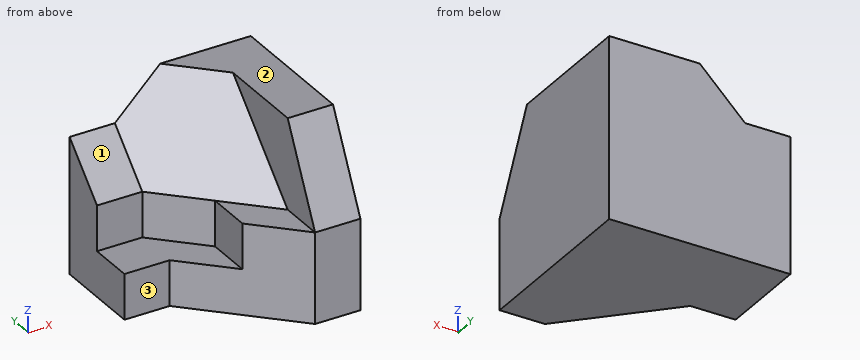
```python
from build123d import *

# Parameters (mm, degrees)
SKETCH1_W            = 40
SKETCH1_H            = 40
BOSS_EXTRUDE1_DEPTH  = 20
CUT_EXTRUDE1_DEPTH   = 20
SKETCH3_W            = 10
SKETCH3_H            = 10
CUT_EXTRUDE2_DEPTH   = 10
BOSS_EXTRUDE2_DEPTH  = 10
BOSS_EXTRUDE3_DEPTH  = 29
BOSS_EXTRUDE4_DEPTH  = 10
CUT_EXTRUDE3_DEPTH   = 10
BOSS_EXTRUDE5_DEPTH  = 10
SKETCH17_W           = 10
SKETCH17_H           = 10
BOSS_EXTRUDE8_DEPTH  = 30
CUT_EXTRUDE4_DEPTH   = 30
CUT_EXTRUDE5_DEPTH   = 10
CUT_EXTRUDE6_DEPTH   = 10
SKETCH21_W           = 5
SKETCH21_H           = 10
BOSS_EXTRUDE9_DEPTH  = 5
CUT_EXTRUDE7_DEPTH   = 5
CUT_EXTRUDE8_DEPTH   = 5
CUT_EXTRUDE9_DEPTH   = 5
BOSS_EXTRUDE10_DEPTH = 5
BOSS_EXTRUDE11_DEPTH = 5
SKETCH27_W           = 20
SKETCH27_H           = 5
BOSS_EXTRUDE12_DEPTH = 40
CUT_EXTRUDE10_DEPTH  = 19


with BuildPart() as part:
    # Sketch1 → Boss-Extrude1 (new body)
    with BuildSketch(Plane.XY):
        with Locations((20, 20)):
            Rectangle(SKETCH1_W, SKETCH1_H)
    extrude(amount=BOSS_EXTRUDE1_DEPTH)

    # Sketch2 → Cut-Extrude1 (cut)
    with BuildSketch(Plane.XY.offset(20)):
        Polygon((0, 0), (30, 0), (10, 20), (0, 20), align=None)
    extrude(amount=-CUT_EXTRUDE1_DEPTH, mode=Mode.SUBTRACT)

    # Sketch3 → Cut-Extrude2 (cut)
    with BuildSketch(Plane.ZY):
        with Locations((15, 25)):
            Rectangle(SKETCH3_W, SKETCH3_H)
    extrude(amount=-CUT_EXTRUDE2_DEPTH, mode=Mode.SUBTRACT)

    # Sketch5 → Boss-Extrude2 (add)
    with BuildSketch(Plane(origin=(40, 0, 0), x_dir=(0, 0, -1), z_dir=(1, 0, 0))):
        Polygon((-20, 40), (-20, 0), (-40, 10), (-40, 40), align=None)
    extrude(amount=-BOSS_EXTRUDE2_DEPTH)

    # Sketch7 → Boss-Extrude3 (add)
    with BuildSketch(Plane.XY.offset(40)):
        Polygon((30, 30), (30, 40), (20, 40), align=None)
    extrude(amount=-BOSS_EXTRUDE3_DEPTH)

    # Sketch8 → Boss-Extrude4 (add)
    with BuildSketch(Plane.ZY):
        Polygon((20, 40), (20, 30), (30, 40), align=None)
    extrude(amount=-BOSS_EXTRUDE4_DEPTH)

    # Sketch9 → Cut-Extrude3 (cut)
    with BuildSketch(Plane.XY.offset(20)):
        Polygon((10, 30), (20, 20), (20, 10), (10, 20), align=None)
    extrude(amount=-CUT_EXTRUDE3_DEPTH, mode=Mode.SUBTRACT)

    # Sketch15 → Boss-Extrude5 (add)
    with BuildSketch(Plane(origin=(6.666666667, 6.666666667, -6.666666667), x_dir=(-0.40824829046386313, -0.40824829046386274, -0.8164965809277261), z_dir=(0.5773502691896262, 0.5773502691896255, -0.5773502691896256))):
        Polygon((-57.154760665, 0), (-57.154760665, 14.142135624), (-32.659863237, 14.142135624), (-32.659863237, -14.142135624), align=None)
    extrude(amount=BOSS_EXTRUDE5_DEPTH)

    # Sketch17 → Boss-Extrude8 (add)
    with BuildSketch(Plane.ZY):
        with Locations((25, 35)):
            Rectangle(SKETCH17_W, SKETCH17_H)
    extrude(amount=-BOSS_EXTRUDE8_DEPTH)

    # Sketch18 → Cut-Extrude4 (cut)
    with BuildSketch(Plane(origin=(0, 40, 0), x_dir=(1, 0, 0), z_dir=(0, 1, 0))):
        Polygon((20, -40), (31.547005384, -34.226497308), (20, -22.679491924), (20, -30), align=None)
    extrude(amount=CUT_EXTRUDE4_DEPTH, mode=Mode.SUBTRACT)

    # Sketch19 → Cut-Extrude5 (cut)
    with BuildSketch(Plane.ZY):
        Polygon((30, 40), (20, 30), (30, 30), align=None)
    extrude(amount=-CUT_EXTRUDE5_DEPTH, mode=Mode.SUBTRACT)

    # Sketch20 → Cut-Extrude6 (cut)
    with BuildSketch(Plane(origin=(6.666666667, 6.666666667, -6.666666667), x_dir=(0.40824829046386324, 0.4082482904638628, 0.816496580927726), z_dir=(-0.5773502691896261, -0.5773502691896254, 0.5773502691896257))):
        Polygon((44.907311951, 7.071067812), (44.907311951, 14.142135624), (32.659863237, 14.142135624), align=None)
    extrude(amount=CUT_EXTRUDE6_DEPTH, mode=Mode.SUBTRACT)

    # Sketch21 → Boss-Extrude9 (add)
    with BuildSketch(Plane(origin=(0, 40, 0), x_dir=(1, 0, 0), z_dir=(0, 1, 0))):
        with Locations((17.5, -35)):
            Rectangle(SKETCH21_W, SKETCH21_H)
    extrude(amount=-BOSS_EXTRUDE9_DEPTH)

    # Sketch22 → Cut-Extrude7 (cut)
    with BuildSketch(Plane(origin=(0, 40, 0), x_dir=(1, 0, 0), z_dir=(0, 1, 0))):
        Polygon((20, -40), (15, -35), (15, -40), align=None)
    extrude(amount=-CUT_EXTRUDE7_DEPTH, mode=Mode.SUBTRACT)

    # Sketch23 → Cut-Extrude8 (cut)
    with BuildSketch(Plane(origin=(6.666666667, 6.666666667, -6.666666667), x_dir=(0.40824829046386324, 0.4082482904638628, 0.816496580927726), z_dir=(-0.5773502691896261, -0.5773502691896254, 0.5773502691896257))):
        Polygon((44.907311951, 14.142135624), (44.907311951, 21.213203436), (32.659863237, 14.142135624), align=None)
    extrude(amount=CUT_EXTRUDE8_DEPTH, mode=Mode.SUBTRACT)


with BuildPart() as cut_extrude8_piece_1:
    # of the separate pieces the step leaves, piece 1, a body of its own (cut_extrude8_pieces)
    add(part.part.solids().sort_by_distance((30, 0, 0))[0])

    # Sketch25 → Boss-Extrude10 (add)
    with BuildSketch(Plane(origin=(0, 40, 0), x_dir=(1, 0, 0), z_dir=(0, 1, 0))):
        Polygon((15, -35), (10, -30), (15, -30), align=None)
    extrude(amount=-BOSS_EXTRUDE10_DEPTH)

    # Sketch26 → Boss-Extrude11 (add)
    with BuildSketch(Plane(origin=(0, 0, 30), x_dir=(-1, 0, 0), z_dir=(0, 0, -1))):
        Polygon((-15, 35), (-10, 40), (-10, 35), align=None)
    extrude(amount=BOSS_EXTRUDE11_DEPTH)

    # Sketch27 → Boss-Extrude12 (add)
    with BuildSketch(Plane(origin=(0, 0, 0), x_dir=(-1, 0, 0), z_dir=(0, 0, -1))):
        with Locations((-30, 37.5)):
            Rectangle(SKETCH27_W, SKETCH27_H)
    extrude(amount=-BOSS_EXTRUDE12_DEPTH)

    # 3DSketch1 → Cut-Extrude10 (cut, along a direction that is not the sketch's normal)
    with BuildSketch(Plane(origin=(10, 30, 20), x_dir=(0.7071067811865477, 0, 0.7071067811865475), z_dir=(0.5773502691896258, 0.5773502691896254, -0.5773502691896261))):
        Polygon((0, 0), (7.071067812, -12.247448714), (21.213203436, -12.247448714), (28.284271247, 0), (14.142135624, 24.494897428), align=None)
    extrude(amount=-CUT_EXTRUDE10_DEPTH, dir=(0, 0, -1), mode=Mode.SUBTRACT)


with BuildPart() as cut_extrude8_piece_2:
    # of the separate pieces the step leaves, piece 2, a body of its own (cut_extrude8_pieces)
    add(part.part.solids().sort_by_distance((10, 30, 30))[0])

    # Sketch24 → Cut-Extrude9 (cut)
    with BuildSketch(Plane(origin=(3.779915321, 3.779915321, -3.779915321), x_dir=(-0.4082482904638635, -0.40824829046386263, -0.816496580927726), z_dir=(0.5773502691896261, 0.5773502691896255, -0.5773502691896258))):
        Polygon((-41.371778045, 14.142135624), (-41.371778045, 15.089479079), (-39.730931049, 14.142135624), align=None)
    extrude(amount=-CUT_EXTRUDE9_DEPTH, mode=Mode.SUBTRACT)


solid = cut_extrude8_piece_1.part
```
For this review, take the finished solid that the model builds, in its own axes (mm). Face numbers are marked on the shaded views. A direction names the side the tool comes from. Coordinates: 2 decimals unless noted, no trailing zeros. Write each loop counter-clockwise with the first axis right and the second up, starting at its lowest first coordinate (ties: lowest second). Pieces come first, ordered by that corner, then holes. Notation, with made-up numbers: (35.5, 23) -> (49.5, 23) arc R23 ccw to (49.5, 58) -> close; hole circle Ø9 at (11.25, 56.25). An arc over 180 degrees is marked (long way). Put each result on its own line as item: value.
Q1. Clearance check with flat-ended pins moving along their axes: pin 1 Ø10 at (x, y) = (8.5, 15.5) entering from +Z; pin 2 Ø3 at (y, z) = (19, 25) entering from -X; pin 3 Ø5 at (x, y) = (25.5, 10) entering from +Z. State where each tip first meets the part, or that it passes through.
From the geometry:
pin 1: stops at z = 10
pin 2: stops at x = 23.88
pin 3: stops at z = 20
Q2. Take a section at B-B, the plane x = 21.5. State the section outline as (y, z) points, then the cut area to 3 significant figures.
From the geometry:
outline: (8.5, 0) -> (40, 0) -> (40, 40) -> (38.5, 40) -> (18.5, 20) -> (8.5, 20) -> close
area: 860 mm2
Q3. Take a section at C-C, the plane z = 3.5. State the section outline as (x, y) points.
From the geometry:
outline: (0, 20) -> (10, 20) -> (30, 0) -> (40, 0) -> (40, 40) -> (0, 40) -> close
Q4. Tool access review of the marked faces 1, 2 and 3: name each direction out of +Z, -Z, +X, -X, +Y, -Y from which nothing blocks a thin tool from reaching the whole face with its end or side.
From the geometry:
face 1: +Z, -X, -Y
face 2: +Z, +X, -X, +Y, -Y
face 3: +Z, -Z, -X, -Y
Q5. Take a section at A-A, the plane y = 12. State the section outline as (x, z) points.
From the geometry:
outline: (18, 0) -> (40, 0) -> (40, 40) -> (30, 40) -> (30, 22) -> (28, 20) -> (20, 20) -> (20, 10) -> (18, 10) -> close
Q6. Take a section at D-D, the plane y = 26. State the section outline as (x, z) points.
From the geometry:
outline: (0, 0) -> (40, 0) -> (40, 40) -> (30, 40) -> (30, 36) -> (14, 20) -> (14, 10) -> (0, 10) -> close
Q7. Wall thickness on L1, parallel to Z at x = 9.5, y = 20.5; L2, parallel to X at y = 10.5, z = 17; L3, parallel to X at y = 5, z = 22.5: over which ranges is each line inside the solid? List them lowest first.
From the geometry:
L1: z = 0 to 10
L2: x = 20 to 40
L3: x = 30 to 40
